Job drawing, mm, ordinate dimensions from the low corner. One solid piece. Round coordinates to 2 decimals unless told otherwise and drop trailing zeros. Write each loop counter-clockwise with the first axis right and the second up, starting at its lowest first coordinate (ties: lowest second). Pieces come first, ordered by that corner, then holes.
1) Flat gauge pins, fed straight in: pin 1 (1.5 mm diameter, centred on y = 1, z = 1, fed in from +X); pin 2 (0.9 mm diameter, centred on y = 1, z = 4.5, fed in from -X); pin 3 (0.9 mm diameter, centred on x = 200.5, y = 1.5, fed in from +Z). Where does each tip first touch, or does it go through?
2) Saw through at C-C (y = 1.55). State how many separate pieces and enclosed holes the cut face has, plus the area to 3 significant figures.
3) Wall check: probe 1 along Z at (x, y) = (161.5, 0.8); probe 2 along X at (y, z) = (0.7, 105). Give the ranges that are in metal, low to high.
4) Saw through at B-B (z = 11). Write the cut outline in (x, y).
5) Saw through at A-A (x = 100). Write the cut outline in (y, z).
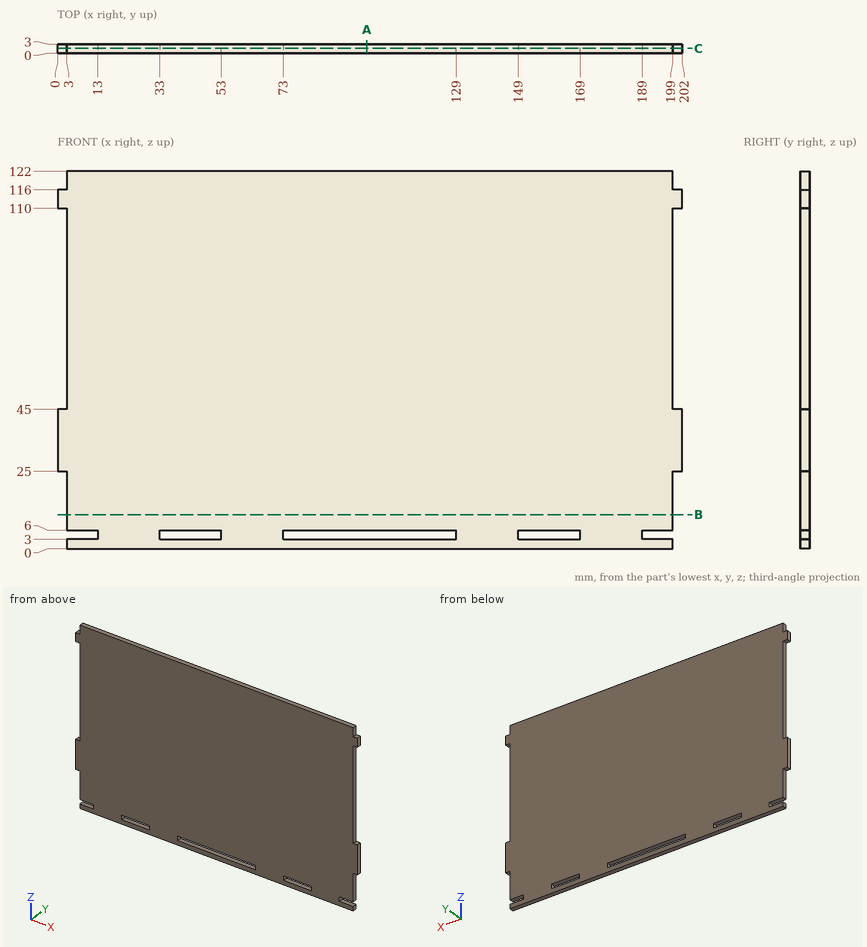
Evaluation:
1. pin 1: stops at x = 199
1. pin 2: stops at x = 13
1. pin 3: stops at z = 116
2. separate pieces: 1
2. enclosed holes: 3
2. area: 23,700 mm2
3. probe 1: z = 0 to 3, 6 to 122
3. probe 2: x = 3 to 199
4. outline: (3, 0) - (199, 0) - (199, 3) - (3, 3) - close
5. outline: (0, 0) - (3, 0) - (3, 3) - (0, 3) - close; (0, 6) - (3, 6) - (3, 122) - (0, 122) - close
